For this review, take the finished solid that the model builds, in its own axes (mm). Face numbers are marked on the shaded views. A direction names the side the tool comes from. Round coordinates to 2 decimals unless told otherwise and drop trailing zeros. Order: outer loops, then holes, each group sorted by start corner. A loop starts at its lowest first (then second) coordinate and runs counter-clockwise, first axis right, second up. Notation, with made-up numbers: M 24.5,28 L 29.5,28 A23 ccw 29.5,63 Z; hole C 84,2.25 d7. An arc over 180 degrees is marked long. Put each result on its own line as item: value.
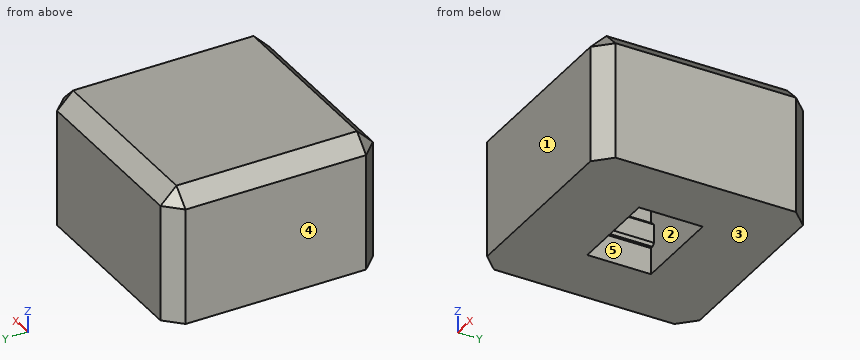
from build123d import *

# Parameters (mm, degrees)
F0_W     = 8
F0_H     = 8
F1_DEPTH = 5
F2_W     = 3.4
F2_H     = 2.4
F3_DEPTH = 3.2
F5_W     = 0.2
F5_H     = 2.4
F6_DEPTH = 0.9
F7_SIZE  = 0.1
F8_SIZE  = 0.6


with BuildPart() as f1:
    # F0 (on Top) → F1 (new body)
    with BuildSketch(Plane.XY):
        Rectangle(F0_W, F0_H)
    extrude(amount=F1_DEPTH)

    # F2 (on Top) → F3 (cut)
    with BuildSketch(Plane.XY):
        Rectangle(F2_W, F2_H)
    extrude(amount=F3_DEPTH, mode=Mode.SUBTRACT)

    # F5 (on offset) → F6 (join)
    with BuildSketch(Plane.XY.offset(1)):
        with Locations((-1.6, 0)):
            Rectangle(F5_W, F5_H)
        with Locations((1.6, 0)):
            Rectangle(F5_W, F5_H)
    extrude(amount=F6_DEPTH)

    # F7
    f7_edges = [f1.edges().sort_by_distance(p)[0] for p in [
        (-1.5, 0, 1),
        (-1.5, 0, 1.9),
        (1.5, 0, 1),
        (1.5, 0, 1.9),
    ]]
    chamfer(f7_edges, length=F7_SIZE)

    # F8
    f8_edges = [f1.edges().sort_by_distance(p)[0] for p in [
        (4, 0, 5),
        (-4, 0, 5),
        (0, -4, 5),
        (0, 4, 5),
        (4, -4, 2.5),
        (4, 4, 2.5),
        (-4, -4, 2.5),
        (-4, 4, 2.5),
    ]]
    chamfer(f8_edges, length=F8_SIZE)


solid = f1.part
(1) For the marked faces 4 and 5, list the 3-axis set-ups (+Z, -Z, +X, -X, +Y, -Y) from which the entire face can be reached by the end or side of a thin tool; tool diameter is ignored.
A:
face 4: +Z, -Z, -X, +Y, -Y
face 5: -Z
(2) Add section C-C on x = -1. Give the boundary of the cut face in (y, z).
A:
outline: M -4,0 L -1.2,0 L -1.2,3.2 L 1.2,3.2 L 1.2,0 L 4,0 L 4,4.4 L 3.4,5 L -3.4,5 L -4,4.4 Z
(3) To check wall thickness, follow L1, parallel to Y at x = 0.5, z = 2.1; L2, parallel to X at y = 0.75, z = 2.8; L3, parallel to X at y = 3.75, z = 2.65. State the ranges of each line that lie inside material, in increasing order.
A:
L1: y = -4 to -1.2, 1.2 to 4
L2: x = -4 to -1.7, 1.7 to 4
L3: x = -3.65 to 3.65
(4) Draft analysis for pull direction Y (two halves, no side actions). For the marked faces 1, 2 and 3, state which applies: released by +Y, released by -Y, zero draft, split by the parting line, or undercut.
A:
face 1: released by -Y
face 2: undercut
face 3: zero draft
(5) Add section A-A on y = 0.25. Give the boundary of the cut face in (x, z).
A:
outline: M -4,0 L -1.7,0 L -1.7,1 L -1.6,1 L -1.5,1.1 L -1.5,1.8 L -1.6,1.9 L -1.7,1.9 L -1.7,3.2 L 1.7,3.2 L 1.7,1.9 L 1.6,1.9 L 1.5,1.8 L 1.5,1.1 L 1.6,1 L 1.7,1 L 1.7,0 L 4,0 L 4,4.4 L 3.4,5 L -3.4,5 L -4,4.4 Z
(6) Add section B-B on z = 1.6. Give the boundary of the cut face in (x, y), then the cut area to 3 significant figures.
A:
outline: M -4,-3.4 L -3.4,-4 L 3.4,-4 L 4,-3.4 L 4,3.4 L 3.4,4 L -3.4,4 L -4,3.4 Z; hole M -1.5,-1.2 L 1.5,-1.2 L 1.5,1.2 L -1.5,1.2 Z
area: 56.1 mm2
